```python
from build123d import *

# Parameters (mm, degrees)
SKETCH1_W                    = 139.7
SKETCH1_H                    = 457.2
SKETCH1_R                    = 50.8
SKETCH1_R_2                  = 5.08
BOSS_EXTRUDE1_DEPTH          = 9.652
SKETCH4_W                    = 10.452383168
SKETCH4_H                    = 4.1148
SKETCH4_W_2                  = 8.864883168
SKETCH4_H_2                  = 6.35
CUT_EXTRUDE1_DEPTH           = 10.652
CHAMFER1_SIZE                = 15.24
CHAMFER1_SIZE2               = 30.48
CHAMFER2_SIZE                = 30.48
CHAMFER2_SIZE2               = 15.24
FILLET2_R                    = 15.24
SKETCH5_W                    = 76.2
SKETCH5_H                    = 9.652
BOSS_EXTRUDE2_DEPTH          = 4.318
F_3_0_3_DIAMETER_HOLE1_D     = 3
F_3_0_3_DIAMETER_HOLE1_DEPTH = 9.652


with BuildPart() as part:
    # Sketch1 → Boss-Extrude1 (new body)
    with BuildSketch(Plane(origin=(0, 0, 0), x_dir=(1, 0, 0), z_dir=(0, 1, 0))):
        with Locations((69.85, 228.6)):
            Rectangle(SKETCH1_W, SKETCH1_H)
        with Locations((63.5, 125.73)):
            Circle(SKETCH1_R, mode=Mode.SUBTRACT)
        with Locations((38.1, 38.1)):
            Circle(SKETCH1_R_2, mode=Mode.SUBTRACT)
        with Locations((38.1, 419.1)):
            Circle(SKETCH1_R_2, mode=Mode.SUBTRACT)
        with Locations((63.5, 331.47)):
            Circle(SKETCH1_R, mode=Mode.SUBTRACT)
        with Locations((38.1, 228.6)):
            Circle(SKETCH1_R_2, mode=Mode.SUBTRACT)
    extrude(amount=BOSS_EXTRUDE1_DEPTH)

    # Sketch4 → Cut-Extrude1 (cut, through all)
    with BuildSketch(Plane(origin=(0, 9.652, 0), x_dir=(1, 0, 0), z_dir=(0, 1, 0))):
        with Locations((5.226191584, 2.0574)):
            Rectangle(SKETCH4_W, SKETCH4_H)
        with Locations((4.432441584, 454.025)):
            Rectangle(SKETCH4_W_2, SKETCH4_H_2)
    extrude(amount=-CUT_EXTRUDE1_DEPTH, mode=Mode.SUBTRACT)

    # Chamfer1
    chamfer1_edges = [part.edges().sort_by_distance(p)[0] for p in [
        (139.7, 4.826, -457.2),
    ]]
    chamfer1_side = [part.faces().sort_by_distance(p)[0] for p in [
        (139.7, 4.826, -228.6),
    ]]
    chamfer(chamfer1_edges, length=CHAMFER1_SIZE, length2=CHAMFER1_SIZE2, reference=chamfer1_side[0])

    # Chamfer2
    chamfer2_edges = [part.edges().sort_by_distance(p)[0] for p in [
        (139.7, 4.826, 0),
    ]]
    chamfer2_side = [part.faces().sort_by_distance(p)[0] for p in [
        (75.076191584, 4.826, 0),
    ]]
    chamfer(chamfer2_edges, length=CHAMFER2_SIZE, length2=CHAMFER2_SIZE2, reference=chamfer2_side[0])

    # Fillet2
    fillet2_edges = [part.edges().sort_by_distance(p)[0] for p in [
        (109.22, 4.826, -457.2),
        (109.22, 4.826, 0),
    ]]
    fillet(fillet2_edges, radius=FILLET2_R)

    # Sketch5 → Boss-Extrude2 (add)
    with BuildSketch(Plane(origin=(139.7, 0, 0), x_dir=(0, 0, -1), z_dir=(1, 0, 0))):
        with Locations((69.85, 4.826)):
            Rectangle(SKETCH5_W, SKETCH5_H)
        with Locations((228.6, 4.826)):
            Rectangle(SKETCH5_W, SKETCH5_H)
        with Locations((387.35, 4.826)):
            Rectangle(SKETCH5_W, SKETCH5_H)
    extrude(amount=BOSS_EXTRUDE2_DEPTH)

    # Ø3.0 (3) Diameter Hole1
    with Locations(Plane(origin=(0, 9.652, 0), x_dir=(1, 0, 0), z_dir=(0, 1, 0))):
        with Locations((101.092, 87.884), (25.4, 87.884), (25.4, 163.576), (101.092, 163.576)):
            f_3_0_3_diameter_hole1 = Hole(F_3_0_3_DIAMETER_HOLE1_D / 2, depth=F_3_0_3_DIAMETER_HOLE1_DEPTH)

    # Mirror1: Ø3.0 (3) Diameter Hole1 across plane
    add(f_3_0_3_diameter_hole1.mirror(Plane.XY.offset(-228.6)), mode=Mode.SUBTRACT)


solid = part.part
```
For this review, take the finished solid that the model builds, in its own axes (mm). A direction names the side the tool comes from. Round coordinates to 2 decimals unless told otherwise and drop trailing zeros. Write each loop counter-clockwise with the first axis right and the second up, starting at its lowest first coordinate (ties: lowest second). Pieces come first, ordered by that corner, then holes. Notation, with made-up numbers: (81.5, 24) - (92.5, 24) arc R35 ccw to (92.5, 60) - close; hole circle Ø10 at (-30.5, -20). An arc over 180 degrees is marked (long way). Put each result on its own line as item: value.
Q1. We need section A-A (z = -125.73). Give the boundary of the cut face in (x, y), and give its area (3 significant figures).
Solved:
outline: (0, 0) - (12.7, 0) - (12.7, 9.65) - (0, 9.65) - close; (114.3, 0) - (139.7, 0) - (139.7, 9.65) - (114.3, 9.65) - close
area: 368 mm2
Q2. We need section B-B (x = 65.5). Give the boundary of the cut face in (y, z).
Solved:
outline: (0, -457.2) - (9.65, -457.2) - (9.65, -382.23) - (0, -382.23) - close; (0, -280.71) - (9.65, -280.71) - (9.65, -176.49) - (0, -176.49) - close; (0, -74.97) - (9.65, -74.97) - (9.65, 0) - (0, 0) - close
Q3. Insertion check: pin 1 Ø4.5 at (y, z) = (3, -2.5) entering from -X; pin 2 Ø6 at (x, z) = (38.1, -38.1) entering from -Y; pin 3 Ø4.5 at (x, y) = (142.5, 6) entering from +Z; pin 4 Ø1.9 at (y, z) = (3, -455) entering from -X. Each pin has a flat end and moves straight along its axis. Give the tip position at first contact, or say it passes through.
Solved:
pin 1: stops at x = 0
pin 2: passes through
pin 3: stops at z = -31.75
pin 4: stops at x = 8.86
Q4. Wall thickness on probe 1 along Z at (x, y) = (65.5, 4.25); probe 2 along Z at (x, y) = (81.5, 3.25); probe 3 along X at (y, z) = (4.5, -100): over which ranges is each line inside the solid? List them lowest first.
Solved:
probe 1: z = -457.2 to -382.23, -280.71 to -176.49, -74.97 to 0
probe 2: z = -457.2 to -378.97, -283.97 to -173.23, -78.23 to 0
probe 3: x = 0 to 19.7, 107.3 to 144.02
Q5. We need section D-D (z = -228.6). Give the boundary of the cut face in (x, y).
Solved:
outline: (0, 0) - (33.02, 0) - (33.02, 9.65) - (0, 9.65) - close; (43.18, 0) - (144.02, 0) - (144.02, 9.65) - (43.18, 9.65) - close
Q6. Machinability: for faces 1 (the face through (139.7, 5, -149)), 2 (the face through (139.7, 5, -23)), 3 (the face through (5, 5, -4.115)), which of the approach directions +Z, -Z, +X, -X, +Y, -Y give a long, thin tool a straight path to every point of the face, cutting with its end or side? Answer none if there is none.
Solved:
face 1: +X, +Y, -Y
face 2: +Z, +X, +Y, -Y
face 3: +Z, -X, +Y, -Y
Q7. We need section C-C (x = 38.1). Give the boundary of the cut face in (y, z), and give its area (3 significant figures).
Solved:
outline: (0, -457.2) - (9.65, -457.2) - (9.65, -424.18) - (0, -424.18) - close; (0, -414.02) - (9.65, -414.02) - (9.65, -375.46) - (0, -375.46) - close; (0, -287.48) - (9.65, -287.48) - (9.65, -233.68) - (0, -233.68) - close; (0, -223.52) - (9.65, -223.52) - (9.65, -169.72) - (0, -169.72) - close; (0, -81.74) - (9.65, -81.74) - (9.65, -43.18) - (0, -43.18) - close; (0, -33.02) - (9.65, -33.02) - (9.65, 0) - (0, 0) - close
area: 2,420 mm2
Q8. Mouldability with a two-part tool opening along Z and no side actions: class faces 4 (the face through (144.018, 5, -228)), 5 (the face through (125.88, 4.76, -448.87)), 6 (the face through (37, 4.76, -33.14)) as released by +Z, released by -Z, zero draft, split by the parting line, or undercut.
Solved:
face 4: zero draft
face 5: released by -Z
face 6: undercut
